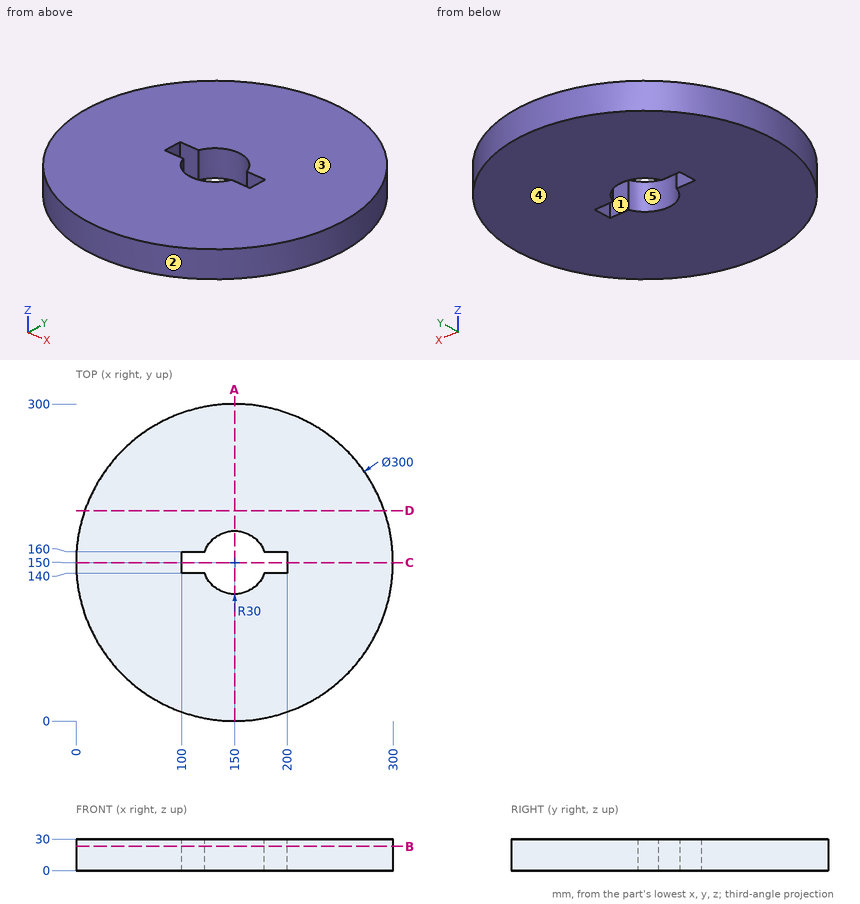
Check sheet for the drawn part. Datum: minimum x, y, z corner. Units: mm. A direction names the side the tool comes from. Round coordinates to 2 decimals unless told otherwise and drop trailing zeros. Order: outer loops, then holes, each group sorted by start corner. A loop starts at its lowest first (then second) coordinate and runs counter-clockwise, first axis right, second up.
(1) Cross-section at C-C, the plane y = 150. Enter the section's corners in (x, z), and give its area (3 significant figures).
(2) Cross-section at D-D, the plane y = 199. Enter the section's corners in (x, z), and give its area (3 significant figures).
(3) Cross-section at A-A, the plane x = 150. Enter the section's corners in (y, z).
(4) Go/stop test with flat-tipped pins: P1, Ø6.5, axis at x = 106.5, z = 10, coming from the +Y side; P2, Ø6, axis at y = 255.5, z = 22, coming from the +X side; P3, Ø3, axis at y = 250.5, z = 7, coming from the -X side. Record where each tip stops, or that it passes through.
(5) Cross-section at B-B, the plane z = 23. Enter the section's corners in (x, y).
(6) Draft check along Y on the marked faces 1, 2 and 3. Enter one of: pulls with the +Y half, pulls with the -Y half, needs draft (parallel to the pull), parting line crosses it, or undercut.
(7) Scan lines: probe 1 along X at (y, z) = (131.5, 10); probe 2 along Y at (x, z) = (102.5, 24.25); probe 3 along Y at (x, z) = (190.5, 3.75). Record each from-to range of solid material in increasing order.
(8) Access from +Z, -Z, +X, -X, +Y, -Y to the whole of each face (thin tool, end or side, straight path). Record for the marked faces 4 and 5.
Check sheet entries:
1. outline: (0, 0) - (100, 0) - (100, 30) - (0, 30) - close; (200, 0) - (300, 0) - (300, 30) - (200, 30) - close
1. area: 6,000 mm2
2. outline: (8.23, 0) - (291.77, 0) - (291.77, 30) - (8.23, 30) - close
2. area: 8,510 mm2
3. outline: (0, 0) - (120, 0) - (120, 30) - (0, 30) - close; (180, 0) - (300, 0) - (300, 30) - (180, 30) - close
4. P1: stops at y = 294.5
4. P2: stops at x = 259.52
4. P3: stops at x = 37.31
5. outline: circle Ø300 at (150, 150); hole (100, 140) - (121.72, 140) arc R30 ccw to (178.28, 140) - (200, 140) - (200, 160) - (178.28, 160) arc R30 ccw to (121.72, 160) - (100, 160) - close
6. face 1: undercut
6. face 2: parting line crosses it
6. face 3: needs draft
7. probe 1: x = 1.15 to 126.38, 173.62 to 298.85
7. probe 2: y = 7.72 to 140, 160 to 292.28
7. probe 3: y = 5.57 to 140, 160 to 294.43
8. face 4: -Z, +X, -X, +Y, -Y
8. face 5: +Z, -Z
